Geometry check sheet. Reference: the model listing, model coordinates, mm. Face numbers are marked on the shaded views. A direction names the side the tool comes from. Round coordinates to 2 decimals unless told otherwise and drop trailing zeros. Order: outer loops, then holes, each group sorted by start corner. A loop starts at its lowest first (then second) coordinate and runs counter-clockwise, first axis right, second up.
(1) Cross-section at A-A on x = -42. Enter the section's corners in (y, z).
(2) Gauge pin test, flat ends, axial feed: P1, Ø3, axis at y = -5, z = 51, coming from the -X side; P2, Ø9.5, axis at x = -45.5, y = -26.5, coming from the +Z side; P3, Ø2, axis at y = -32, z = 41, coming from the +X side; P4, Ø9.5, axis at x = -49.5, z = 52, coming from the -Y side. Record the tip position at first contact, or that the pin passes through.
(3) Cross-section at C-C on z = 36.5. Enter the section's corners in (x, y), and give its area (3 significant figures).
(4) Set-up check for the marked faces 1, 2 and 3: record each of +Z, -Z, +X, -X, +Y, -Y from which the full face is reachable in a straight line by a thin tool's end or side.
(5) Cross-section at D-D on z = 15.5. Enter the section's corners in (x, y), and give its area (3 significant figures).
(6) Cross-section at B-B on y = -14. Enter the section's corners in (x, z).
(7) Thickness scan on L1, parallel to Y at x = -65.5, z = 32; L2, parallel to Z at x = -46, y = -34; L3, parallel to Z at x = -60, y = -16. Record the ranges inside material, lowest first.
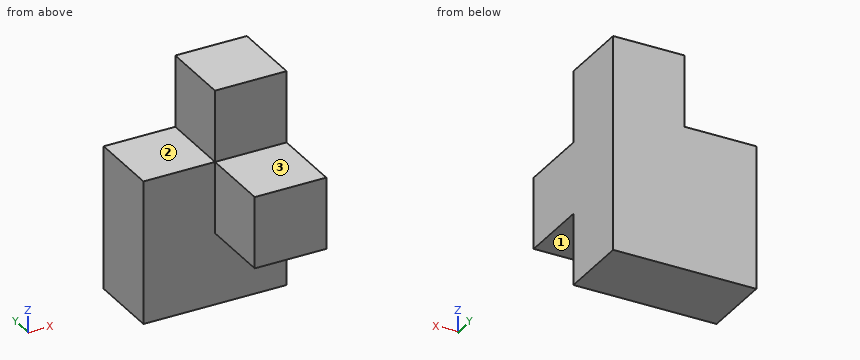
from build123d import *

# Parameters (mm, degrees)
F0_W     = 19.05
F0_H     = 19.05
F1_DEPTH = 19.05
F2_W     = 19.05
F2_H     = 19.05
F3_DEPTH = 38.1
F4_ANGLE = 180


with BuildPart() as f1:
    # F0 (on Front) → F1 (new body)
    with BuildSketch(Plane.XZ):
        with Locations((-28.575, 47.625)):
            Rectangle(F0_W, F0_H)
        Polygon((-19.05, 38.1), (-38.1, 38.1), (-38.1, 0), (0, 0), (0, 38.1), align=None)
    extrude(amount=-F1_DEPTH)

    # F2 (on Front) → F3 (join)
    with BuildSketch(Plane.XZ):
        with Locations((-28.575, 28.575)):
            Rectangle(F2_W, F2_H)
    extrude(amount=-F3_DEPTH)


with BuildPart() as f1_1:
    # F4: moved
    add(f1.part.rotate(Axis((-38.1, 0, 28.575), (0, 0, -1)), F4_ANGLE))


solid = f1_1.part
Found:
1. outline: (-38.1, 19.05) - (-19.05, 19.05) - (-19.05, 0) - (0, 0) - (0, 57.15) - (-19.05, 57.15) - (-19.05, 38.1) - (-38.1, 38.1) - close
2. P1: stops at x = -57.15
2. P2: stops at z = 38.1
2. P3: passes through
2. P4: stops at y = -19.05
3. outline: (-76.2, -19.05) - (-57.15, -19.05) - (-57.15, -38.1) - (-38.1, -38.1) - (-38.1, 0) - (-76.2, 0) - close
3. area: 1,090 mm2
4. face 1: -Z, +X, -X, -Y
4. face 2: +Z, -X, +Y, -Y
4. face 3: +Z, +X, -X, -Y
5. outline: (-76.2, -19.05) - (-38.1, -19.05) - (-38.1, 0) - (-76.2, 0) - close
5. area: 726 mm2
6. outline: (-76.2, 0) - (-38.1, 0) - (-38.1, 57.15) - (-57.15, 57.15) - (-57.15, 38.1) - (-76.2, 38.1) - close
7. L1: y = -19.05 to 0
7. L2: z = 19.05 to 38.1
7. L3: z = 0 to 38.1
